Could you check a few things on this model? Use its own coordinates, in mm. Coordinates: 2 decimals unless noted, no trailing zeros. Loops run counter-clockwise (first coordinate to the right, second up) from the corner with the lowest first, then second, coordinate; pieces in that order, holes last.
1) If I drill on line 1 along Z through (x, y) = (2, 4); line 2 along Y through (x, z) = (2.75, 0); line 3 along Y through (x, z) = (0.5, -1), over which ranges is the centre line in solid material (lowest first)?
2) Imagine slicing it at C-C on y = -2.5. Please give me the cut outline in (x, z).
3) Imagine slicing it at D-D on z = 10. Please give me the cut outline in (x, y), plus the area to 3 significant figures.
4) Thinking about a two-plate mould opening in Y: for faces 1 (the face through (6.35, -2, 3)), 2 (the face through (3.131, -10.14, -5.274)), 3 (the face through (3.13, -3.35, 0.74)), which applies, released by +Y, released by -Y, zero draft, split by the parting line, or undercut?
5) Imagine slicing it at A-A on y = 0. Please give me the cut outline in (x, z), plus the area to 3 significant figures.
6) Will these pins go through, and if not, where does the flat tip stop? P1, Ø6, axis at y = 0, z = 0, coming from the -X side; P2, Ø3, axis at x = 5, y = 3, coming from the -Z side; P3, Ø1.5, axis at x = 0.5, z = -9, coming from the +Y side; P4, Ø1.5, axis at x = 5.5, y = 4, coming from the +Z side.
```python
from build123d import *

# Parameters (mm, degrees)
SKETCH1_R           = 11.43
SKETCH1_R_2         = 3.429
BOSS_EXTRUDE1_DEPTH = 6.35
CUT_EXTRUDE1_DEPTH  = 14.986


with BuildPart() as part:
    # Sketch1 → Boss-Extrude1 (new body)
    with BuildSketch(Plane(origin=(0, 0, 0), x_dir=(0, 0, -1), z_dir=(1, 0, 0))):
        Circle(SKETCH1_R)
        Circle(SKETCH1_R_2, mode=Mode.SUBTRACT)
    extrude(amount=BOSS_EXTRUDE1_DEPTH)

    # Sketch2 → Cut-Extrude1 (cut)
    with BuildSketch(Plane(origin=(0, 0, 0), x_dir=(1, 0, 0), z_dir=(0, 1, 0))):
        with BuildLine():
            ThreePointArc((5.55625, 0), (5.070783, 1.440957453), (3.812326951, 2.294377022))
            Line((3.812326951, 2.294377022), (3.175, 0))
            Line((3.175, 0), (3.812326951, -2.294377022))
            ThreePointArc((3.812326951, -2.294377022), (5.070783, -1.440957453), (5.55625, 0))
        make_face()
        with BuildLine():
            Line((3.175, 0), (3.812326951, 2.294377022))
            ThreePointArc((3.812326951, 2.294377022), (3.175, 2.38125), (2.537673049, 2.294377022))
            Line((2.537673049, 2.294377022), (3.175, 0))
        make_face()
        with BuildLine():
            Line((3.812326951, -2.294377022), (3.175, 0))
            Line((3.175, 0), (2.537673049, -2.294377022))
            ThreePointArc((2.537673049, -2.294377022), (3.175, -2.38125), (3.812326951, -2.294377022))
        make_face()
        with BuildLine():
            Line((2.537673049, -2.294377022), (3.175, 0))
            Line((3.175, 0), (2.537673049, 2.294377022))
            ThreePointArc((2.537673049, 2.294377022), (0.79375, 0), (2.537673049, -2.294377022))
        make_face()
    extrude(amount=CUT_EXTRUDE1_DEPTH, mode=Mode.SUBTRACT)


solid = part.part
```
Filled in:
1. line 1: z = -10.71 to -2.07, 2.07 to 10.71
1. line 2: y = -11.43 to -3.43
1. line 3: y = -11.39 to -3.28, 3.28 to 11.39
2. outline: (0, -11.15) - (6.35, -11.15) - (6.35, -2.35) - (0, -2.35) - close; (0, 2.35) - (6.35, 2.35) - (6.35, 11.15) - (0, 11.15) - close
3. outline: (0, -5.54) - (6.35, -5.54) - (6.35, 5.54) - (0, 5.54) - close
3. area: 70.3 mm2
4. face 1: zero draft
4. face 2: split by the parting line
4. face 3: undercut
5. outline: (0, -11.43) - (6.35, -11.43) - (6.35, -3.43) - (0, -3.43) - close; (0, 3.43) - (6.35, 3.43) - (6.35, 11.43) - (0, 11.43) - close
5. area: 102 mm2
6. P1: passes through
6. P2: stops at z = -11.33
6. P3: stops at y = 7.91
6. P4: stops at z = 10.96
